Autodesk Inventor part; units mm, degrees
ref_plane "YZ Plane" through (0, 0, 0) normal (1, 0, 0) x (0, 1, 0)
ref_plane "XZ Plane" through (0, 0, 0) normal (0, 1, 0) x (-1, 0, 0)
ref_plane "XY Plane" through (0, 0, 0) normal (0, 0, 1) x (1, 0, 0)
sketch "Sketch1" plane through (0, 0, 0) normal (0, 0, 1) x (1, 0, 0)
  line L0 (-20.05, 15.1) -> (20.05, 15.1)
  line L1 (20.05, 15.1) -> (20.05, -15.1)
  line L2 (20.05, -15.1) -> (-20.05, -15.1)
  line L3 (-20.05, -15.1) -> (-20.05, 15.1)
  line L4 (-20.05, 15.1) -> (20.05, -15.1) construction
  line L5 (20.05, 15.1) -> (-20.05, -15.1) construction
  arc A0 (-20.05, -4.5) -> (-20.05, 4.5) centre (-22.85, 0) ccw
  line L6 (-22.85, 0) -> (-17.55, 0) construction
  line L7 (-17.55, 0) -> (0, 0) construction
  dimension "d0" = 40.1
  dimension "d1" = 30.2
  dimension "d2" = 2.5
  dimension "d3" = 9
extrude "Extrusion1" add sketch "Sketch1" against normal blind 6.6 contours L0 L1 L2 L3 A0
sketch "Sketch2" plane through (0, 0, -6.6) normal (0, 0, -1) x (-1, 0, 0)
  line L0 (-15, -0.1) -> (15, -0.1)
  line L1 (15, -0.1) -> (15, -15.1)
  line L2 (15, -15.1) -> (-15, -15.1)
  line L3 (-15, -15.1) -> (-15, -0.1)
  line L4 (-15, -0.1) -> (15, -15.1) construction
  line L5 (15, -0.1) -> (-15, -15.1) construction
  line L6 (-20.05, -15.1) -> (20.05, -15.1)
  point P0 (0, 0)
  point P1 (0, -7.6)
  point P2 (0, -15.1)
  dimension "d6" = 30
  dimension "d7" = 15
extrude "Extrusion2" add sketch "Sketch2" along normal blind 25
sketch "Sketch3" plane through (0, 0, 0) normal (0, 1, 0) x (-1, 0, 0)
  line L0 (0, 0) -> (0, 43)
  line L1 (0, 0) -> (11, 0)
  line L2 (11, 0) -> (11, 4.5)
  line L3 (11, 4.5) -> (14.35, 4.5)
  line L4 (14.35, 4.5) -> (14.35, 11.1)
  line L5 (14.35, 11.1) -> (13.85, 11.1)
  line L6 (13.85, 11.1) -> (13.85, 12.1)
  line L7 (13.85, 12.1) -> (15, 12.1)
  line L8 (15, 12.1) -> (15, 15.45)
  line L9 (15, 15.45) -> (13.5, 16.95)
  line L10 (13.5, 16.95) -> (13.5, 23)
  line L11 (13.5, 23) -> (15, 23)
  line L12 (15, 23) -> (15, 37)
  line L13 (15, 37) -> (20, 37)
  line L14 (20, 37) -> (20, 42)
  line L15 (20, 43) -> (0, 43) construction
  arc A0 (20, 42) -> (0, 43) centre (0, -157.5) ccw
  line L16 (20, 42) -> (20, 43) construction
  dimension "d10" = 22
  dimension "d11" = 4.5
  dimension "d12" = 28.7
  dimension "d13" = 6.6
  dimension "d14" = 3.35
  dimension "d15" = 30
  dimension "d16" = 0.5
  dimension "d17" = 1
  dimension "d18" = 27
  dimension "d19" = 30
  dimension "d20" = 40
  dimension "d21" = 6
  dimension "d22" = 20
  dimension "d23" = 43
  dimension "d24" = 45
  dimension "d26" = 1
revolve "Revolution1" add sketch "Sketch3" angle 360 about axis through (0, 0, 0) along (0, 0, 1)
fillet "Fillet1" radius 2 3 edges at (20, 0, 42) (20, 0, 37) (15, 0, 37)
fillet "Fillet2" radius 1 4 edges at (20.05, -15.1, -3.3) (20.05, 15.1, -3.3) (-20.05, 15.1, -3.3) (-20.05, -15.1, -3.3)
sketch "Sketch4" plane through (-15, -0.1, -6.6) normal (0, 1, 0) x (1, 0, 0)
  line L0 (30, 0) -> (0, 0)
  line L1 (30, 0) -> (30, 25)
  line L2 (0, 25) -> (30, 25)
  line L3 (0, 0) -> (0, 25)
  line L4 (30, 0) -> (30, 25)
  line L5 (30, 11.5) -> (28.5, 0)
  line L6 (0, 11.5) -> (1.5, 0)
  line L7 (0, 25) -> (30, 25) construction
  line L8 (15, 25) -> (15, 0) construction
  point P0 (15, -6.6)
  dimension "d29" = 27
  dimension "d30" = 11.5
extrude "Extrusion3" cut sketch "Sketch4" against normal through all contours L0 L5 L1 | L0 L3 L6
properties part number "emergency-button" material "ABS Plastic"
Input: part model. Units: mm. Frame: model coordinates. A direction names the side the tool comes from. Coordinates: 2 decimals unless noted, no trailing zeros. Loops run counter-clockwise (first coordinate to the right, second up) from the corner with the lowest first, then second, coordinate; pieces in that order, holes last. Notation, with made-up numbers: (36.25, 31) -> (58.25, 31) arc R26 ccw to (58.25, 56) -> close; hole circle Ø4 at (31, 82). An arc over 180 degrees is marked (long way). Write each question's results on one line, items separated by ' | '. Start each with the question number.
Q1. Section B-B, the plane z = 2. Return the cut outline in (x, y), plus the area to 3 significant figures.
Q2. Reachability of faces 4 (the cylindrical face through (-7.714, -12.1, 7.846)), 5 (the flat face through (15, -8, -25)), 6 (the cylindrical face through (-19.076, -6.007, 39.599)), 7 (the flat face through (0, 15.1, -3)), 8 (the flat face through (-15, -7, -25)) from +Z, -Z, +X, -X, +Y, -Y: full face, straight path, thin tool, end or side. Return the list, or none.
Q3. Pin query (flat end, axial travel): pin 1 (9 mm diameter, centred on x = -2.5, y = 5, fed in from -Z); pin 2 (4 mm diameter, centred on y = -11, z = -25.5, fed in from +X); pin 3 (11 mm diameter, centred on y = -5, z = -27.5, fed in from -X); pin 4 (8.5 mm diameter, centred on x = 1.5, y = 0.5, fed in from +Z). Return the tip coordinate at first contact, or that it passes through.
Q4. Section C-C, the plane z = -13. Return the cut outline in (x, y), plus the area to 3 significant figures.
Q5. Ray query, line 1 (Z direction, x = 12, y = 8.5); line 2 (Z direction, x = -3, y = 14.5); line 3 (Y direction, x = -12, z = -20). Return the intervals inside material, ascending. Write a range as from..to.
Q6. Pull-direction query (Z, two-part tool) for faces 1 (the flat face through (3, 11, 4.5)), 2 (the flat face through (0, -15.1, -16)), 3 (the flat face through (-4.4, 13.3, 12.1)); classes: released by +Z, released by -Z, zero draft, split by the parting line, or undercut.
Q7. Section A-A, the plane z = 29. Return the cut outline in (x, y).
Found:
1) outline: circle Ø22 at (0, 0) | area: 380 mm2
2) face 4: none | face 5: -Z, +X, +Y, -Y | face 6: +Z | face 7: -Z, +X, -X, +Y | face 8: -Z, -X, +Y, -Y
3) pin 1: z = -6.6 | pin 2: x = 15 | pin 3: x = -15 | pin 4: z = 43
4) outline: (-14.33, -15.1) -> (14.33, -15.1) -> (14.33, -0.1) -> (-14.33, -0.1) -> close | area: 430 mm2
5) line 1: -6.6..0, 12.1..15.74, 23..42.46 | line 2: -6.6..0, 12.1..15.64, 23..42.45 | line 3: -15.1..-0.1
6) face 1: undercut | face 2: zero draft | face 3: undercut
7) outline: circle Ø30 at (0, 0)
